Autodesk Inventor part; units mm, degrees
ref_plane "YZ Plane" through (0, 0, 0) normal (1, 0, 0) x (0, 1, 0)
ref_plane "XZ Plane" through (0, 0, 0) normal (0, 1, 0) x (-1, 0, 0)
ref_plane "XY Plane" through (0, 0, 0) normal (0, 0, 1) x (1, 0, 0)
sketch "Sketch1" plane through (0, 0, 0) normal (0, 0, 1) x (1, 0, 0)
  line L0 (-23.6233, -6.7963) -> (65.3767, -6.7963)
  line L1 (65.3767, -6.7963) -> (65.3767, 82.2037)
  line L2 (65.3767, 82.2037) -> (-23.6233, 82.2037)
  line L3 (-23.6233, 82.2037) -> (-23.6233, -6.7963)
  line L4 (-23.6233, 93.2037) -> (65.3767, 93.2037)
  line L5 (65.3767, 93.2037) -> (65.3767, 182.2037)
  line L6 (65.3767, 182.2037) -> (-23.6233, 182.2037)
  line L7 (-23.6233, 182.2037) -> (-23.6233, 93.2037)
  line L8 (-23.6233, 193.2037) -> (65.3767, 193.2037)
  line L9 (65.3767, 193.2037) -> (65.3767, 282.2037)
  line L10 (65.3767, 282.2037) -> (-23.6233, 282.2037)
  line L11 (-23.6233, 282.2037) -> (-23.6233, 193.2037)
  line L12 (-23.6233, 293.2037) -> (65.3767, 293.2037)
  line L13 (65.3767, 293.2037) -> (65.3767, 382.2037)
  line L14 (65.3767, 382.2037) -> (-23.6233, 382.2037)
  line L15 (-23.6233, 382.2037) -> (-23.6233, 293.2037)
  line L16 (76.3767, -6.7963) -> (165.3767, -6.7963)
  line L17 (165.3767, -6.7963) -> (165.3767, 82.2037)
  line L18 (165.3767, 82.2037) -> (76.3767, 82.2037)
  line L19 (76.3767, 82.2037) -> (76.3767, -6.7963)
  line L20 (76.3767, 93.2037) -> (165.3767, 93.2037)
  line L21 (165.3767, 93.2037) -> (165.3767, 182.2037)
  line L22 (165.3767, 182.2037) -> (76.3767, 182.2037)
  line L23 (76.3767, 182.2037) -> (76.3767, 93.2037)
  line L24 (76.3767, 193.2037) -> (165.3767, 193.2037)
  line L25 (165.3767, 193.2037) -> (165.3767, 282.2037)
  line L26 (165.3767, 282.2037) -> (76.3767, 282.2037)
  line L27 (76.3767, 282.2037) -> (76.3767, 193.2037)
  line L28 (76.3767, 293.2037) -> (165.3767, 293.2037)
  line L29 (165.3767, 293.2037) -> (165.3767, 382.2037)
  line L30 (165.3767, 382.2037) -> (76.3767, 382.2037)
  line L31 (76.3767, 382.2037) -> (76.3767, 293.2037)
  line L32 (176.3767, -6.7963) -> (265.3767, -6.7963)
  line L33 (265.3767, -6.7963) -> (265.3767, 82.2037)
  line L34 (265.3767, 82.2037) -> (176.3767, 82.2037)
  line L35 (176.3767, 82.2037) -> (176.3767, -6.7963)
  line L36 (176.3767, 93.2037) -> (265.3767, 93.2037)
  line L37 (265.3767, 93.2037) -> (265.3767, 182.2037)
  line L38 (265.3767, 182.2037) -> (176.3767, 182.2037)
  line L39 (176.3767, 182.2037) -> (176.3767, 93.2037)
  line L40 (176.3767, 193.2037) -> (265.3767, 193.2037)
  line L41 (265.3767, 193.2037) -> (265.3767, 282.2037)
  line L42 (265.3767, 282.2037) -> (176.3767, 282.2037)
  line L43 (176.3767, 282.2037) -> (176.3767, 193.2037)
  line L44 (176.3767, 293.2037) -> (265.3767, 293.2037)
  line L45 (265.3767, 293.2037) -> (265.3767, 382.2037)
  line L46 (265.3767, 382.2037) -> (176.3767, 382.2037)
  line L47 (176.3767, 382.2037) -> (176.3767, 293.2037)
  line L48 (276.3767, -6.7963) -> (365.3767, -6.7963)
  line L49 (365.3767, -6.7963) -> (365.3767, 82.2037)
  line L50 (365.3767, 82.2037) -> (276.3767, 82.2037)
  line L51 (276.3767, 82.2037) -> (276.3767, -6.7963)
  line L52 (276.3767, 93.2037) -> (365.3767, 93.2037)
  line L53 (365.3767, 93.2037) -> (365.3767, 182.2037)
  line L54 (365.3767, 182.2037) -> (276.3767, 182.2037)
  line L55 (276.3767, 182.2037) -> (276.3767, 93.2037)
  line L56 (276.3767, 193.2037) -> (365.3767, 193.2037)
  line L57 (365.3767, 193.2037) -> (365.3767, 282.2037)
  line L58 (365.3767, 282.2037) -> (276.3767, 282.2037)
  line L59 (276.3767, 282.2037) -> (276.3767, 193.2037)
  line L60 (276.3767, 293.2037) -> (365.3767, 293.2037)
  line L61 (365.3767, 293.2037) -> (365.3767, 382.2037)
  line L62 (365.3767, 382.2037) -> (276.3767, 382.2037)
  line L63 (276.3767, 382.2037) -> (276.3767, 293.2037)
  circle A0 centre (-33.6233, -16.7963) radius 4
  arc A1 (-42.1947, -11.6455) -> (-33.6233, 19.2592) centre (-93.6233, 19.2592) ccw
  arc A2 (2.4322, -16.7963) -> (-28.4725, -25.3677) centre (2.4322, -76.7963) ccw
  arc A3 (-42.1947, -11.6455) -> (-28.4725, -25.3677) centre (-33.6233, -16.7963) ccw
  arc A4 (375.3767, 19.2592) -> (383.9481, -11.6455) centre (435.3767, 19.2592) ccw
  circle A5 centre (375.3767, -16.7963) radius 4
  arc A6 (370.2259, -25.3677) -> (383.9481, -11.6455) centre (375.3767, -16.7963) ccw
  arc A7 (370.2259, -25.3677) -> (339.3212, -16.7963) centre (339.3212, -76.7963) ccw
  arc A8 (339.3212, 392.2037) -> (370.2259, 400.7751) centre (339.3212, 452.2037) ccw
  circle A9 centre (375.3767, 392.2037) radius 4
  arc A10 (383.9481, 387.0529) -> (370.2259, 400.7751) centre (375.3767, 392.2037) ccw
  arc A11 (383.9481, 387.0529) -> (375.3767, 356.1482) centre (435.3767, 356.1482) ccw
  arc A12 (-33.6233, 356.1482) -> (-42.1947, 387.0529) centre (-93.6233, 356.1482) ccw
  circle A13 centre (-33.6233, 392.2037) radius 4
  arc A14 (-28.4725, 400.7751) -> (-42.1947, 387.0529) centre (-33.6233, 392.2037) ccw
  arc A15 (-28.4725, 400.7751) -> (2.4322, 392.2037) centre (2.4322, 452.2037) ccw
  line L64 (2.4322, -16.7963) -> (339.3212, -16.7963)
  line L65 (375.3767, 19.2592) -> (375.3767, 356.1482)
  line L66 (-33.6233, 356.1482) -> (-33.6233, 19.2592)
  line L67 (339.3212, 392.2037) -> (2.4322, 392.2037)
  point P0 (0, 0)
  point P1 (0, 100)
  point P2 (0, 200)
  point P3 (0, 300)
  point P4 (100, 0)
  point P5 (100, 100)
  point P6 (100, 200)
  point P7 (100, 300)
  point P8 (200, 0)
  point P9 (200, 100)
  point P10 (200, 200)
  point P11 (200, 300)
  point P12 (300, 0)
  point P13 (300, 100)
  point P14 (300, 200)
  point P15 (300, 300)
  point P16 (170.8767, 187.7037)
  dimension "d0" = 89
  dimension "d1" = 89
  dimension "d4" = 100
  dimension "d7" = 100
  dimension "d10" = 8
  dimension "d11" = 10
  dimension "d12" = 10
  dimension "d17" = 60
  dimension "d18" = 60
  dimension "d21" = 360
extrude "Extrusion1" add sketch "Sketch1" along normal blind 5
sketch "Sketch2" plane through (0, 0, 5) normal (0, 0, 1) x (1, 0, 0)
  line L0 (165.3767, 182.2037) -> (165.3767, 93.2037)
  line L1 (265.3767, 193.2037) -> (176.3767, 193.2037)
  line L2 (165.3767, 182.2037) -> (176.3767, 182.2037)
  line L3 (176.3767, 182.2037) -> (176.3767, 193.2037)
  line L4 (176.3767, 193.2037) -> (165.3767, 193.2037)
  line L5 (165.3767, 193.2037) -> (165.3767, 182.2037)
  point P0 (0, 0)
  point P1 (170.8767, 187.7037)
properties part number "b-base"
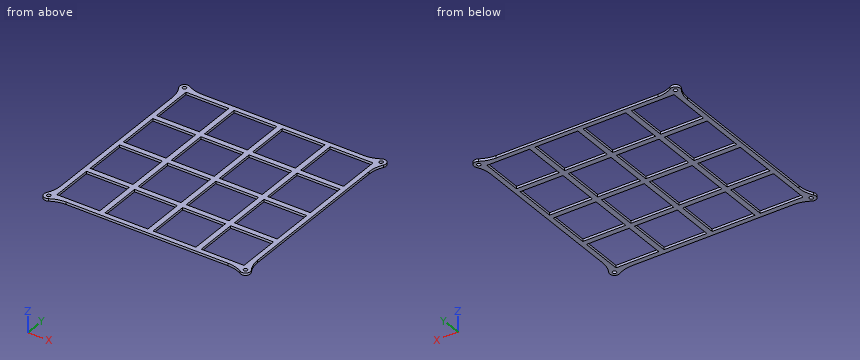
The model under review builds one solid part; all positions refer to its coordinate system, in mm. Give positions to 0.01 mm unless a question says otherwise; leave off trailing zeros. Write each loop counter-clockwise with the first axis right and the second up, starting at its lowest first coordinate (ties: lowest second). Pieces come first, ordered by that corner, then holes. Notation, with made-up numbers: M 51,47.25 L 59,47.25 A15 cw 59,68.25 Z; hole C 71,43.25 d6. An arc over 180 degrees is marked long. One line per question, with ' | ' between items. Start each with the question number.
Item 1: We need section C-C on z = 1.7. Give the number of separate pieces and of enclosed holes in the cut face, plus the area to 3 significant figures.
Item 2: We need section A-A on y = 43. Write out the cut boundary in (x, z).
Item 3: For pin 1 (2.5 mm diameter, centred on y = 155.5, z = 3.5, fed in from -X); pin 2 (2.5 mm diameter, centred on y = 259.5, z = 1.5, fed in from +X); pin 3 (1.5 mm diameter, centred on x = 304, z = 2.5, fed in from +Y), all flat-tipped, find the tip position at first contact; note any pin that passes through.
Item 4: We need section B-B on x = 237. Write out the cut boundary in (y, z), plus the area to 3 significant figures.
Item 5: Wall thickness on line 1 (Y direction, x = 86, z = 1.6); line 2 (X direction, y = 108, z = 4.6); line 3 (Y direction, x = -13.5, z = 4.8): over which ranges is each line inside the solid? List them lowest first. Write a range as from..to.
Results found:
1) separate pieces: 1 | enclosed holes: 20 | area: 41,700 mm2
2) outline: M -33.62,0 L -23.62,0 L -23.62,5 L -33.62,5 Z; M 65.38,0 L 76.38,0 L 76.38,5 L 65.38,5 Z; M 165.38,0 L 176.38,0 L 176.38,5 L 165.38,5 Z; M 265.38,0 L 276.38,0 L 276.38,5 L 265.38,5 Z; M 365.38,0 L 375.38,0 L 375.38,5 L 365.38,5 Z
3) pin 1: stops at x = -33.62 | pin 2: stops at x = 375.38 | pin 3: stops at y = 392.2
4) outline: M -16.8,0 L -6.8,0 L -6.8,5 L -16.8,5 Z; M 82.2,0 L 93.2,0 L 93.2,5 L 82.2,5 Z; M 182.2,0 L 193.2,0 L 193.2,5 L 182.2,5 Z; M 282.2,0 L 293.2,0 L 293.2,5 L 282.2,5 Z; M 382.2,0 L 392.2,0 L 392.2,5 L 382.2,5 Z | area: 265 mm2
5) line 1: y = -16.8..-6.8, 82.2..93.2, 182.2..193.2, 282.2..293.2, 382.2..392.2 | line 2: x = -33.62..-23.62, 65.38..76.38, 165.38..176.38, 265.38..276.38, 365.38..375.38 | line 3: y = -18.95..-6.8, 82.2..93.2, 182.2..193.2, 282.2..293.2, 382.2..394.36
